Could you check a few things on this model? Use its own coordinates, in mm. Face numbers are marked on the shaded views. A direction names the side the tool comes from. Coordinates: 2 decimals unless noted, no trailing zeros. Loops run counter-clockwise (first coordinate to the right, second up) from the corner with the lowest first, then second, coordinate; pieces in that order, holes last.
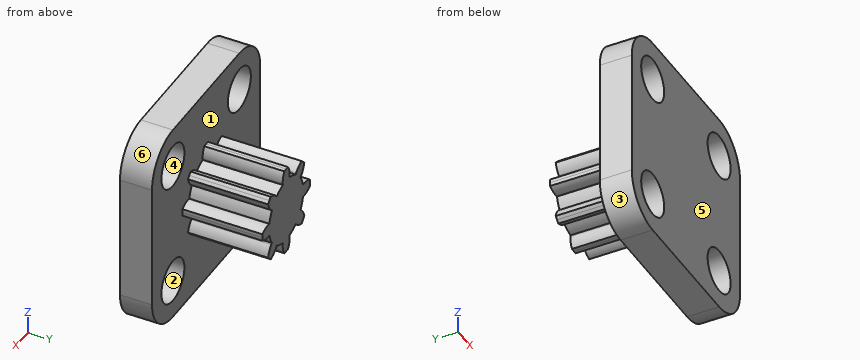
Autodesk Inventor part; units mm, degrees
ref_plane "YZ Plane" through (0, 0, 0) normal (1, 0, 0) x (0, 1, 0)
ref_plane "XZ Plane" through (0, 0, 0) normal (0, 1, 0) x (-1, 0, 0)
ref_plane "XY Plane" through (0, 0, 0) normal (0, 0, 1) x (1, 0, 0)
sketch "Sketch1" plane through (0, 0, 0) normal (0, 1, 0) x (-1, 0, 0)
  line L0 (7.955, -7.955) -> (-7.955, -7.955)
  line L1 (-7.955, -7.955) -> (-7.955, 7.955)
  line L2 (-7.955, 7.955) -> (7.955, 7.955)
  line L3 (7.955, 7.955) -> (7.955, -7.955)
  circle A0 centre (7.955, -7.955) radius 5
  circle A1 centre (7.955, -7.955) radius 2.75
  line L4 (0, 0) -> (4.4409, 0)
  line L5 (0, 0) -> (0, 4.5835)
  circle A2 centre (7.955, 7.955) radius 5
  circle A3 centre (7.955, 7.955) radius 2.75
  circle A4 centre (-7.955, -7.955) radius 5
  circle A5 centre (-7.955, -7.955) radius 2.75
  circle A6 centre (-7.955, 7.955) radius 2.75
  circle A7 centre (-7.955, 7.955) radius 5
  line L6 (12.955, 7.955) -> (12.955, -7.955)
  line L7 (7.955, -12.955) -> (-7.955, -12.955)
  line L8 (7.955, 12.955) -> (-7.955, 12.955)
  line L9 (-12.955, 7.955) -> (-12.955, -7.955)
  dimension "d0" = 11.25
  dimension "d1" = 10
  dimension "d2" = 5.5
extrude "Extrusion1" add sketch "Sketch1" along normal blind 4 contours A4 L1 A5 L0 | A4 L1 A7 L2 A2 L3 A0 L0 | L0 A0 L7 A4 | L0 A5 L1 A4 | A0 L3 A1 L0 | L0 A1 L3 A0 | A4 L9 A7 L1 | L3 A2 L6 A0 | A7 L2 A6 L1 | L1 A6 L2 A7 | A2 L2 A3 L3 | L3 A3 L2 A2 | A7 L8 A2 L2
sketch "Sketch2" plane through (0, 4, 0) normal (0, 1, 0) x (1, 0, 0)
  arc A0 (0.45, 5.6822) -> (0, 5.7) centre (0, 0) ccw
  arc A1 (0.7683, 4.9406) -> (0, 5) centre (0, 0) ccw construction
  arc A2 (0.8, 4.0214) -> (0, 4.1002) centre (0, 0) ccw
  line L0 (0.839, 4.2174) -> (0.8, 4.0214)
  arc A3 (0.839, 4.2174) -> (0, 4.3) centre (0, 0) ccw construction
  arc A4 (0.839, 4.2174) -> (0.45, 5.6822) centre (-1.6581, 4.3383) ccw
  line L1 (-0.839, 4.2174) -> (-0.8, 4.0214)
  arc A5 (-0.45, 5.6822) -> (-0.839, 4.2174) centre (1.6581, 4.3383) ccw
  arc A6 (0, 5) -> (0.7683, 4.9406) centre (0, 0) ccw construction
  arc A7 (0, 5.7) -> (0.45, 5.6822) centre (0, 0) ccw
  arc A8 (0, 4.3) -> (0.839, 4.2174) centre (0, 0) ccw construction
  arc A9 (0, 4.1002) -> (0.8, 4.0214) centre (0, 0) ccw
  dimension "d12" = 10
  dimension "d13" = 2.5
  dimension "d14" = 0.7
  dimension "d15" = 0.7
  dimension "d16" = 0.1998
  dimension "d17" = 0.8
  dimension "d18" = 0.45
extrude "Extrusion2" add sketch "Sketch2" along normal blind 10 contours A9 A2
extrude "Extrusion3" add sketch "Sketch2" along normal blind 10 contours A4 L0 A2 A9 L1 A5 A7 A0
pattern_circular "Circular Pattern1" count 8 over 360 about axis through (0, 4, 0) along (0, 1, 0) of "Extrusion2", "Extrusion3"
properties part number "Carrier_V2_CPY" material "Polystyrene"
(1) Imagine slicing it at C-C, the plane y = 2. Write out the boundary of the cut face in (x, z) (3 decimals), and give its area (3 significant figures).
Answers:
outline: (-12.955, -7.955) arc R5 ccw to (-7.955, -12.955) - (7.955, -12.955) arc R5 ccw to (12.955, -7.955) - (12.955, 7.955) arc R5 ccw to (7.955, 12.955) - (-7.955, 12.955) arc R5 ccw to (-12.955, 7.955) - close; hole circle Ø5.5 at (-7.955, -7.955); hole circle Ø5.5 at (-7.955, 7.955); hole circle Ø5.5 at (7.955, -7.955); hole circle Ø5.5 at (7.955, 7.955)
area: 555 mm2
(2) I need wall thicknesses on probe 1 along X at (y, z) = (1.75, 10); probe 2 along Z at (x, y) = (-7, 1) (3 decimals); probe 3 along Y at (x, z) = (2.75, 8.5). Which ranges of each line are inside material? Lowest first, please.
Answers:
probe 1: x = -12.52 to -9.79, -6.12 to 6.12, 9.79 to 12.52
probe 2: z = -12.955 to -10.534, -5.376 to 5.376, 10.534 to 12.955
probe 3: y = 0 to 4
(3) Which directions (+Z, -Z, +X, -X, +Y, -Y) give clear straight access to the entire face, cutting with the end or side of a thin tool? Please do the marked faces 1 and 2.
Answers:
face 1: +Y
face 2: +Y, -Y
(4) For pin 1 (2 mm diameter, centred on x = -8, z = -1, fed in from +Y); pin 2 (6 mm diameter, centred on x = 7.5, z = -1, fed in from +Y); pin 3 (5 mm diameter, centred on x = -7.955, z = 7.955, fed in from +Y); pin 4 (2 mm diameter, centred on y = 10.5, z = -2.5, fed in from -X), each with a flat end and sliding along its axis, tell me the tip position at first contact or that it passes through.
Answers:
pin 1: stops at y = 4
pin 2: stops at y = 14
pin 3: passes through
pin 4: stops at x = -4.28
(5) Imagine slicing it at D-D, the plane z = 11.75. Write out the boundary of the cut face in (x, y).
Answers:
outline: (-11.21, 0) - (11.21, 0) - (11.21, 4) - (-11.21, 4) - close
(6) Imagine slicing it at A-A, the plane z = -7. Write out the boundary of the cut face in (x, y) (3 decimals).
Answers:
outline: (-12.955, 0) - (-10.534, 0) - (-10.534, 4) - (-12.955, 4) - close; (-5.376, 0) - (5.376, 0) - (5.376, 4) - (-5.376, 4) - close; (10.534, 0) - (12.955, 0) - (12.955, 4) - (10.534, 4) - close
(7) Imagine slicing it at B-B, the plane x = -8.5. Write out the boundary of the cut face in (y, z), and give its area (3 significant figures).
Answers:
outline: (0, -12.93) - (4, -12.93) - (4, -10.65) - (0, -10.65) - close; (0, -5.26) - (4, -5.26) - (4, 5.26) - (0, 5.26) - close; (0, 10.65) - (4, 10.65) - (4, 12.93) - (0, 12.93) - close
area: 60.3 mm2
(8) We'd pull the mould along Z, two halves only. Please class the marked faces 3, 4, 5 and 6: +Z half, -Z half, draft (parallel to the pull), parting line (faces both ways), or undercut.
Answers:
face 3: -Z half
face 4: undercut
face 5: draft
face 6: +Z half
